Source: three-view drawing plus pictorial views. Frame: mm from the lowest corner of the part. A direction names the side the tool comes from. Coordinates: 2 decimals unless noted, no trailing zeros. Write each loop counter-clockwise with the first axis right and the second up, starting at its lowest first coordinate (ties: lowest second). Pieces come first, ordered by that corner, then holes. Notation, with made-up numbers: M 41,-24.5 L 89,-24.5 A8 ccw 89,-11.5 Z; hole C 67,85.5 d10. An arc over 180 degrees is marked long. Use CSV: the item, a comma, the result in double quotes.
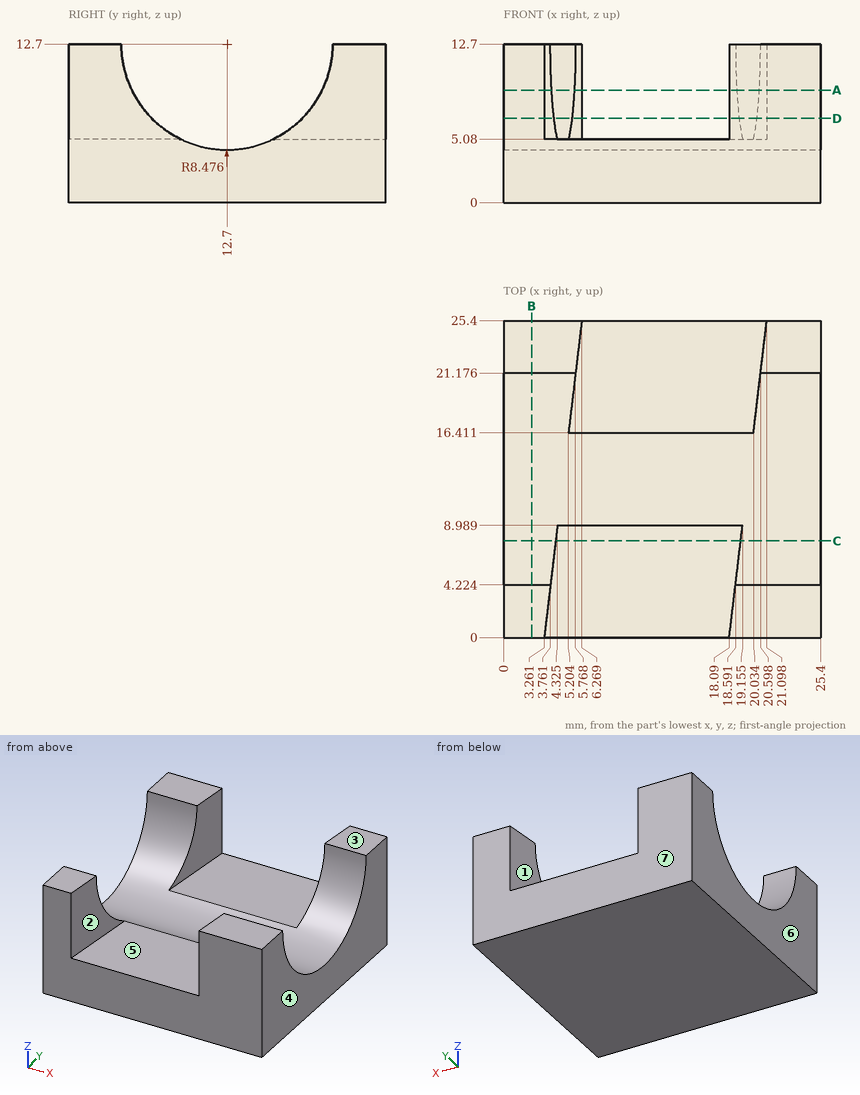
1. Mould query, pull axis X, two halves, no side actions, for the marked faces 4, 5, 6 and 7. Classes: pulls with the +X half, pulls with the -X half, needs draft (parallel to the pull), parting line crosses it, or undercut.
Resolved:
face 4,"pulls with the +X half"
face 5,"undercut"
face 6,"pulls with the -X half"
face 7,"needs draft"
2. Section B-B (x = 2.25). Return loops of the section in (y, z) (1 decimal), then the cut area to 3 significant figures.
Resolved:
outline,"M 0,0 L 25.4,0 L 25.4,12.7 L 21.2,12.7 A8.5 cw 4.2,12.7 L 0,12.7 Z"
area,"210 mm^2"
3. Access query for the marked faces 1, 2 and 3. Directions: +Z, -Z, +X, -X, +Y, -Y. A direction counts if a zero-diameter tool reaches every point of the face in a straight line with its end or side. Return the directions, or none.
Resolved:
face 1,"+Z, +Y"
face 2,"+Z, -Y"
face 3,"+Z, +X, -X, +Y, -Y"
4. Section C-C (y = 7.75). Return loops of the section in (x, z), then the cut area to 3 significant figures.
Resolved:
outline,"M 0,0 L 25.4,0 L 25.4,5.82 L 19.01,5.82 L 19.01,5.08 L 4.18,5.08 L 4.18,5.82 L 0,5.82 Z"
area,"137 mm^2"
5. Material intervals for line 1 (Z direction, x = 13.5, y = 20.5); line 2 (Y direction, x = 22, z = 7.5) (1 decimal); line 3 (X direction, y = 21.5, z = 11), sorted ascending. Write a range as [from, to].
Resolved:
line 1,"z = [0, 5.08]"
line 2,"y = [0, 6], [19.4, 25.4]"
line 3,"x = [0, 5.81], [20.64, 25.4]"
6. Section A-A (z = 9). Return loops of the section in (x, y) (1 decimal).
Resolved:
outline,"M 0,0 L 3.3,0 L 3.9,5.1 L 0,5.1 Z; M 0,20.3 L 5.7,20.3 L 6.3,25.4 L 0,25.4 Z; M 18.1,0 L 25.4,0 L 25.4,5.1 L 18.7,5.1 Z; M 20.5,20.3 L 25.4,20.3 L 25.4,25.4 L 21.1,25.4 Z"
7. Section D-D (z = 6.75). State how many separate pieces and enclosed holes the cut face has, then the cut area to 3 significant figures.
Resolved:
separate pieces,"4"
enclosed holes,"0"
area,"141 mm^2"
8. Contact query for flat-ended pins moving along their axis: pin 1 Ø3 at (x, y) = (10, 12) entering from +Z (1 decimal); pin 2 Ø3 at (x, y) = (9.5, 5.5) entering from +Z; pin 3 Ø2 at (x, y) = (3, 6.5) entering from +Z. Output: stop coordinate, or through.
Resolved:
pin 1,"stops at z = 4.5"
pin 2,"stops at z = 5.08"
pin 3,"stops at z = 8.23"
